Here's how the part is built. I have some questions about the finished solid (model axes, mm). A direction names the side the tool comes from. Coordinates: 2 decimals unless noted, no trailing zeros. Write each loop counter-clockwise with the first axis right and the second up, starting at its lowest first coordinate (ties: lowest second). Pieces come first, ordered by that corner, then holes. Notation, with made-up numbers: (70, -17) -> (91, -17) arc R13 ccw to (91, 7) -> close; hole circle Ø9 at (71, 41). An arc over 180 degrees is marked (long way). Put each result on its own line as item: value.
```python
from build123d import *

# Parameters (mm, degrees)
SKETCH1_R            = 36.5
BOSS_EXTRUDE1_DEPTH  = 5
SKETCH4_W            = 3
SKETCH4_H            = 6
SKETCH4_W_2          = 6
SKETCH4_H_2          = 3
BOSS_EXTRUDE4_DEPTH  = 15
SKETCH6_R            = 2
BOSS_EXTRUDE6_DEPTH  = 2.5
SKETCH7_R            = 2
BOSS_EXTRUDE8_DEPTH  = 2.5
BOSS_EXTRUDE9_START  = -2.5
SKETCH9_R            = 2
BOSS_EXTRUDE9_DEPTH  = 2.5
BOSS_EXTRUDE10_START = -2.5
SKETCH10_R           = 2
BOSS_EXTRUDE10_DEPTH = 2.5


with BuildPart() as part:
    # Sketch1 → Boss-Extrude1 (new body)
    with BuildSketch(Plane.XY):
        Circle(SKETCH1_R)
    extrude(amount=BOSS_EXTRUDE1_DEPTH)

    # Sketch4 → Boss-Extrude4 (add)
    with BuildSketch(Plane(origin=(0, 0, 0), x_dir=(-1, 0, 0), z_dir=(0, 0, -1))):
        with Locations((-34.75, 0)):
            Rectangle(SKETCH4_W, SKETCH4_H)
        with Locations((34.75, 0)):
            Rectangle(SKETCH4_W, SKETCH4_H)
        with Locations((0, 34.75)):
            Rectangle(SKETCH4_W_2, SKETCH4_H_2)
        with Locations((0, -34.75)):
            Rectangle(SKETCH4_W_2, SKETCH4_H_2)
    extrude(amount=BOSS_EXTRUDE4_DEPTH)

    # Sketch6 → Boss-Extrude6 (add)
    with BuildSketch(Plane(origin=(36.25, 0, 0), x_dir=(0, 0, -1), z_dir=(1, 0, 0))):
        with Locations((13, 0)):
            Circle(SKETCH6_R)
    extrude(amount=BOSS_EXTRUDE6_DEPTH)

    # Sketch7 → Boss-Extrude8 (add)
    with BuildSketch(Plane(origin=(0, -36.25, -62.5), x_dir=(1, 0, 0), z_dir=(0, 1, 0))):
        with Locations(Location((0, -49.5, 0), (0, 0, 270))):
            Circle(SKETCH7_R)
    extrude(amount=-BOSS_EXTRUDE8_DEPTH)

    # Sketch9 → Boss-Extrude9 (add)
    with BuildSketch(Plane(origin=(-36.25, 0, -62.5), x_dir=(0, 0, -1), z_dir=(1, 0, 0)).offset(BOSS_EXTRUDE9_START)):
        with Locations((-49.5, 0)):
            Circle(SKETCH9_R)
    extrude(amount=BOSS_EXTRUDE9_DEPTH)

    # Sketch10 → Boss-Extrude10 (add)
    with BuildSketch(Plane(origin=(0, 36.25, 0), x_dir=(-1, 0, 0), z_dir=(0, -1, 0)).offset(BOSS_EXTRUDE10_START)):
        with Locations(Location((0, 13, 0), (0, 0, 270))):
            Circle(SKETCH10_R)
    extrude(amount=BOSS_EXTRUDE10_DEPTH)


solid = part.part
```
Item 1: Imagine slicing it at D-D on y = 10.5. Write out the boundary of the cut face in (x, z), then the cut area to 3 significant figures.
Output:
outline: (-34.96, 0) -> (34.96, 0) -> (34.96, 5) -> (-34.96, 5) -> close
area: 350 mm²
Item 2: For P1, Ø1, axis at x = 21, y = -4, coming from the -Z side; P2, Ø4, axis at y = 23.5, z = 1.5, coming from the -X side; P3, Ø2.5, axis at x = 35, z = -11, coming from the +Y side, each with a flat end and sliding along its axis, tell me the tip position at first contact or that it passes through.
Output:
P1: stops at z = 0
P2: stops at x = -29.5
P3: stops at y = 3
Item 3: Imagine slicing it at B-B on z = -8. Write out the boundary of the cut face in (x, y).
Output:
outline: (-36.25, -3) -> (-33.25, -3) -> (-33.25, 3) -> (-36.25, 3) -> close; (-3, -36.25) -> (3, -36.25) -> (3, -33.25) -> (-3, -33.25) -> close; (-3, 33.25) -> (3, 33.25) -> (3, 36.25) -> (-3, 36.25) -> close; (33.25, -3) -> (36.25, -3) -> (36.25, 3) -> (33.25, 3) -> close
Item 4: If we mould it in two halves opening along Y, with no side actions, what happens to faces 1 (the flat face through (0, 33.25, -7)), 2 (the flat face through (0, 38.75, -13)), 3 (the flat face through (-3, 35, -7))? For each: released by +Y, released by -Y, zero draft, split by the parting line, or undercut.
Output:
face 1: undercut
face 2: released by +Y
face 3: zero draft
Item 5: Which directions (+Z, -Z, +X, -X, +Y, -Y) give clear straight access to the entire face, cutting with the end or side of a thin tool? Please do faces 4 (the cylindrical face through (-37.5, -1.2, -11.4)), 5 (the flat face through (-35, 3, -7)), 6 (the flat face through (3, 35, -7)).
Output:
face 4: -X
face 5: -Z, +X, -X, +Y
face 6: -Z, +X, +Y, -Y
Item 6: Imagine slicing it at C-C on x = 1. Write out the boundary of the cut face in (y, z), then the cut area to 3 significant figures.
Output:
outline: (-38.75, -14.73) -> (-36.25, -14.73) -> (-36.25, -15) -> (-33.25, -15) -> (-33.25, 0) -> (33.25, 0) -> (33.25, -15) -> (36.25, -15) -> (36.25, -14.73) -> (38.75, -14.73) -> (38.75, -11.27) -> (36.25, -11.27) -> (36.25, 0) -> (36.49, 0) -> (36.49, 5) -> (-36.49, 5) -> (-36.49, 0) -> (-36.25, 0) -> (-36.25, -11.27) -> (-38.75, -11.27) -> close
area: 472 mm²
Item 7: Please list where these lines run through material, in increasing order: line 1 along Z through (x, y) = (17, -31.5); line 2 along X through (y, z) = (2.5, -6); line 3 along Y through (x, z) = (-35, -0.75). Write a range as from..to.
Output:
line 1: z = 0..5
line 2: x = -36.25..-33.25, 33.25..36.25
line 3: y = -3..3
Item 8: Imagine slicing it at A-A on z = -13. State how many separate pieces and enclosed holes the cut face has, then the cut area to 3 significant figures.
Output:
separate pieces: 4
enclosed holes: 0
area: 112 mm²
